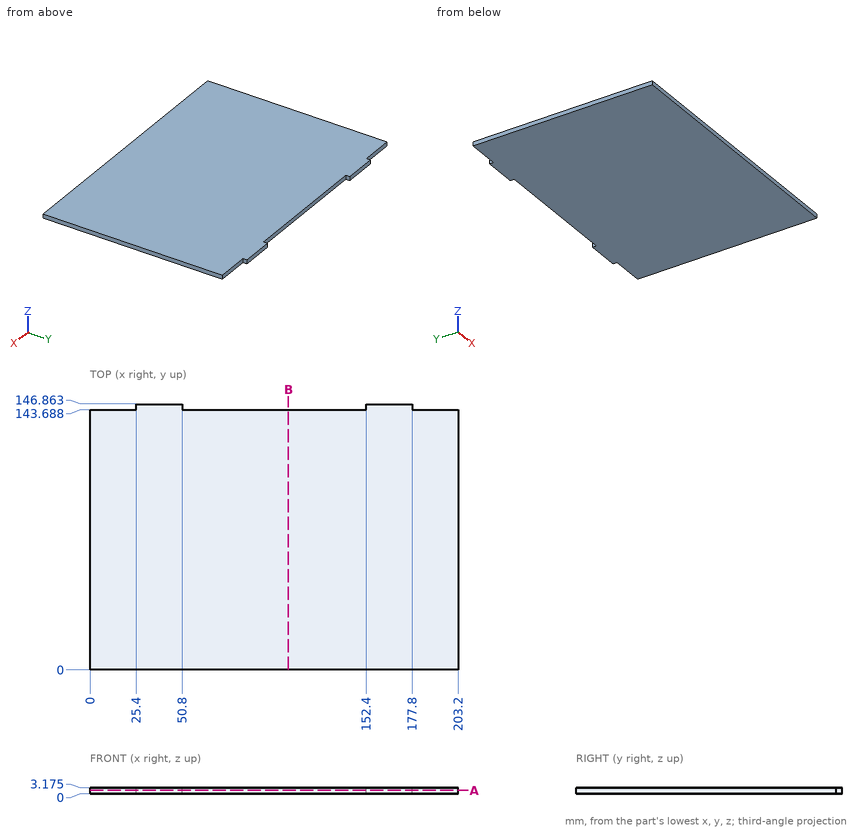
Design review of the part shown in the three views and the two pictorial views. Dimensions are in mm from the part's minimum x, y and z. Coordinates: 2 decimals unless noted, no trailing zeros. Write each loop counter-clockwise with the first axis right and the second up, starting at its lowest first coordinate (ties: lowest second). Pieces come first, ordered by that corner, then holes.
1) We need section B-B on x = 109.5. State the section outline as (y, z) points (1 decimal), then the cut area to 3 significant figures.
2) To check wall thickness, follow probe 1 along Y at (x, z) = (98.5, 1.05). State the ranges of the line that lie inside material, in increasing order.
3) Clearance check with flat-ended pins moving along their axes: pin 1 Ø3 at (x, y) = (101.5, 39) entering from -Z; pin 2 Ø1 at (y, z) = (145, 1.5) entering from -X. State where each tip first meets the part, or that it passes through.
4) We need section A-A on z = 1.85. State the section outline as (x, y) points.
Answer list:
1. outline: (0, 0) - (143.7, 0) - (143.7, 3.2) - (0, 3.2) - close
1. area: 456 mm2
2. probe 1: y = 0 to 143.69
3. pin 1: stops at z = 0
3. pin 2: stops at x = 25.4
4. outline: (0, 0) - (203.2, 0) - (203.2, 143.69) - (177.8, 143.69) - (177.8, 146.86) - (152.4, 146.86) - (152.4, 143.69) - (50.8, 143.69) - (50.8, 146.86) - (25.4, 146.86) - (25.4, 143.69) - (0, 143.69) - close
